from build123d import *

# Parameters (mm, degrees)
F0_W     = 88.9
F0_H     = 50.8
F0_R     = 4.7625
F1_DEPTH = 19.05
F2_SIZE  = 5.08
F3_SIZE  = 0.8128
F4_SIZE  = 1.6002


with BuildPart() as f1:
    # F0 (on Top) → F1 (new body)
    with BuildSketch(Plane.XY):
        Rectangle(F0_W, F0_H)
        with Locations((-25.4, -12.7)):
            Circle(F0_R, mode=Mode.SUBTRACT)
        with Locations((25.4, -12.7)):
            Circle(F0_R, mode=Mode.SUBTRACT)
        with Locations((-25.4, 12.7)):
            Circle(F0_R, mode=Mode.SUBTRACT)
        with Locations((25.4, 12.7)):
            Circle(F0_R, mode=Mode.SUBTRACT)
    extrude(amount=F1_DEPTH)

    # F2
    f2_edges = [f1.edges().sort_by_distance(p)[0] for p in [
        (44.45, -25.4, 9.525),
        (44.45, 25.4, 9.525),
        (-44.45, 25.4, 9.525),
        (-44.45, -25.4, 9.525),
    ]]
    chamfer(f2_edges, length=F2_SIZE)

    # F3
    f3_edges = [f1.edges().sort_by_distance(p)[0] for p in [
        (-30.1625, 12.7, 19.05),
        (-30.1625, 12.7, 0),
        (20.6375, 12.7, 19.05),
        (20.6375, 12.7, 0),
        (20.6375, -12.7, 19.05),
        (20.6375, -12.7, 0),
        (-30.1625, -12.7, 19.05),
        (-30.1625, -12.7, 0),
    ]]
    chamfer(f3_edges, length=F3_SIZE)

    # F4
    f4_edges = [f1.edges().sort_by_distance(p)[0] for p in [
        (0, -25.4, 19.05),
        (-44.45, 0, 19.05),
        (0, 25.4, 19.05),
        (-44.45, 0, 0),
        (0, -25.4, 0),
        (44.45, 0, 19.05),
        (44.45, 0, 0),
        (0, 25.4, 0),
    ]]
    chamfer(f4_edges, length=F4_SIZE)


solid = f1.part
The model under review builds one solid part; all positions refer to its coordinate system, in mm. Give positions to 0.01 mm unless a question says otherwise; leave off trailing zeros. Loops run counter-clockwise (first coordinate to the right, second up) from the corner with the lowest first, then second, coordinate; pieces in that order, holes last. Notation, with made-up numbers: (-37.75, 8.5) -> (-5.75, 8.5) arc R33 cw to (-5.75, 36.5) -> close; hole circle Ø3 at (46, 5). An arc over 180 degrees is marked (long way). Answer as a JSON object with one key per item and string values. Group by question number.
Q1. Wall thickness on line 1 along Y through (x, z) = (-25.4, 10.75); line 2 along X through (y, z) = (10, 16.25); line 3 along X through (y, z) = (-10.5, 15): over which ranges is each line inside the solid? List them lowest first.
Q2. Take a section at A-A (y = 12.7). Write out the cut boundary in (x, z), plus the area to 3 significant figures.
Q3. Take a section at B-B (x = 25.4). Write out the cut boundary in (y, z).
Q4. Take a section at C-C (z = 5.75). State how many separate pieces and enclosed holes the cut face has, plus the area to 3 significant figures.
Q5. Draft analysis for pull direction Y (two halves, no side actions). For faces 1 (the flat face through (43.6, -0.3, 18.3)), 2 (the cylindrical face through (27.598, 8.475, 9.403)), 3 (the flat face through (-1, -25.4, 9)), state which applies: pulls with the +Y half, pulls with the -Y half, needs draft (parallel to the pull), parting line crosses it, or undercut.
Answer below:
{
 "1": {"line 1": "y = -25.4 to -17.46, -7.94 to 7.94, 17.46 to 25.4", "line 2": "x = -44.45 to -29.32, -21.48 to 21.48, 29.32 to 44.45", "line 3": "x = -44.45 to -29.62, -21.18 to 21.18, 29.62 to 44.45"},
 "2": {"outline": "(-44.45, 1.6) -> (-42.85, 0) -> (-30.98, 0) -> (-30.16, 0.81) -> (-30.16, 18.24) -> (-30.98, 19.05) -> (-42.85, 19.05) -> (-44.45, 17.45) -> close; (-20.64, 0.81) -> (-19.82, 0) -> (19.82, 0) -> (20.64, 0.81) -> (20.64, 18.24) -> (19.82, 19.05) -> (-19.82, 19.05) -> (-20.64, 18.24) -> close; (30.16, 0.81) -> (30.98, 0) -> (42.85, 0) -> (44.45, 1.6) -> (44.45, 17.45) -> (42.85, 19.05) -> (30.98, 19.05) -> (30.16, 18.24) -> close", "area": "1,320 mm2"},
 "3": {"outline": "(-25.4, 1.6) -> (-23.8, 0) -> (-18.28, 0) -> (-17.46, 0.81) -> (-17.46, 18.24) -> (-18.28, 19.05) -> (-23.8, 19.05) -> (-25.4, 17.45) -> close; (-7.94, 0.81) -> (-7.12, 0) -> (7.12, 0) -> (7.94, 0.81) -> (7.94, 18.24) -> (7.12, 19.05) -> (-7.12, 19.05) -> (-7.94, 18.24) -> close; (17.46, 0.81) -> (18.28, 0) -> (23.8, 0) -> (25.4, 1.6) -> (25.4, 17.45) -> (23.8, 19.05) -> (18.28, 19.05) -> (17.46, 18.24) -> close"},
 "4": {"separate pieces": "1", "enclosed holes": "4", "area": "4,180 mm2"},
 "5": {"face 1": "needs draft", "face 2": "undercut", "face 3": "pulls with the -Y half"}
}
